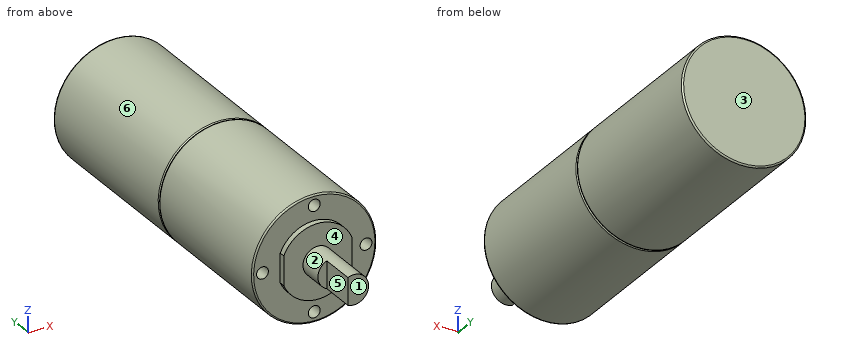
```python
from build123d import *

# Parameters (mm, degrees)
CROQUIS1_R              = 21
SALIENTE_EXTRUIR1_DEPTH = 60
REDONDEO1_R             = 0.5
SALIENTE_EXTRUIR2_START = 53
CROQUIS2_R              = 21
SALIENTE_EXTRUIR2_DEPTH = 53
REDONDEO2_R             = 0.5
SALIENTE_EXTRUIR3_DEPTH = 2
CROQUIS4_R              = 5
SALIENTE_EXTRUIR4_DEPTH = 20.5
CORTAR_EXTRUIR1_START   = -12
CORTAR_EXTRUIR1_DEPTH   = 12
CROQUIS6_R              = 2
CORTAR_EXTRUIR2_DEPTH   = 5


with BuildPart() as part:
    # Croquis1 → Saliente-Extruir1 (new body)
    with BuildSketch(Plane(origin=(0, 0, 0), x_dir=(1, 0, 0), z_dir=(0, 1, 0))):
        with Locations(Location((0, 0, 0), (0, 0, 270))):
            Circle(CROQUIS1_R)
    extrude(amount=SALIENTE_EXTRUIR1_DEPTH)

    # Redondeo1
    redondeo1_edges = [part.edges().sort_by_distance(p)[0] for p in [
        (0, 0, -21),
        (0, 60, -21),
    ]]
    fillet(redondeo1_edges, radius=REDONDEO1_R)

    # Croquis2 → Saliente-Extruir2 (add)
    with BuildSketch(Plane.XZ.offset(SALIENTE_EXTRUIR2_START)):
        with Locations(Location((0, 0, 0), (0, 0, 90))):
            Circle(CROQUIS2_R)
    extrude(amount=-SALIENTE_EXTRUIR2_DEPTH)

    # Redondeo2
    redondeo2_edges = [part.edges().sort_by_distance(p)[0] for p in [
        (0, 0, -21),
        (0, -53, -21),
    ]]
    fillet(redondeo2_edges, radius=REDONDEO2_R - 0.0001)  # a hair under: the kernel refuses the full size

    # Croquis3 → Saliente-Extruir3 (add)
    with BuildSketch(Plane.XZ.offset(53)):
        with BuildLine():
            Line((11.5, -4.898979486), (11.5, 4.898979486))
            ThreePointArc((11.5, 4.898979486), (0, 12.5), (-11.5, 4.898979486))
            Line((-11.5, 4.898979486), (-11.5, -4.898979486))
            ThreePointArc((-11.5, -4.898979486), (0, -12.5), (11.5, -4.898979486))
        make_face()
    extrude(amount=SALIENTE_EXTRUIR3_DEPTH)

    # Croquis4 → Saliente-Extruir4 (add)
    with BuildSketch(Plane.XZ.offset(55)):
        with Locations(Location((0, 0, 0), (0, 0, 270))):
            Circle(CROQUIS4_R)
    extrude(amount=SALIENTE_EXTRUIR4_DEPTH)

    # Croquis5 → Cortar-Extruir1 (cut)
    with BuildSketch(Plane.XZ.offset(75.5).offset(CORTAR_EXTRUIR1_START)):
        with BuildLine():
            Line((-2, 4.582575695), (-2, -4.582575695))
            ThreePointArc((-2, -4.582575695), (-5, 0), (-2, 4.582575695))
        make_face()
    extrude(amount=CORTAR_EXTRUIR1_DEPTH, mode=Mode.SUBTRACT)

    # Croquis6 → Cortar-Extruir2 (cut)
    with BuildSketch(Plane.XZ.offset(53)):
        with Locations(Location((-17.5, 0, 0), (0, 0, 270))):
            Circle(CROQUIS6_R)
        with Locations(Location((0, 17.5, 0), (0, 0, 270))):
            Circle(CROQUIS6_R)
        with Locations(Location((17.5, 0, 0), (0, 0, 270))):
            Circle(CROQUIS6_R)
        with Locations(Location((0, -17.5, 0), (0, 0, 270))):
            Circle(CROQUIS6_R)
    extrude(amount=-CORTAR_EXTRUIR2_DEPTH, mode=Mode.SUBTRACT)


solid = part.part
```
Could you check a few things on this model? Use its own coordinates, in mm. Face numbers are marked on the shaded views. A direction names the side the tool comes from. Round coordinates to 2 decimals unless told otherwise and drop trailing zeros. Order: outer loops, then holes, each group sorted by start corner. A loop starts at its lowest first (then second) coordinate and runs counter-clockwise, first axis right, second up. Notation, with made-up numbers: M 60.5,46 L 81.5,46 A29 cw 81.5,78 Z; hole C 38,22.25 d5. An arc over 180 degrees is marked long. One line per question, with ' | ' between items. Start each with the question number.
(1) Please list where these lines run through material, in increasing order: line 1 along X through (y, z) = (-49.65, 0); line 2 along Y through (x, z) = (-12, -16); line 3 along Y through (x, z) = (0, -11.5).
(2) For the marked faces 4, 5 and 6, which set-ups out of +Z, -Z, +X, -X, +Y, -Y let a thin tool reach every point of the face, with its end or its side?
(3) Suppose I cut it at D-D on y = -59. List the corners of the cut face in (x, z) for me.
(4) For P1, Ø1.5, axis at x = -16, y = -24.5, coming from the -Z side; P2, Ø4.5, axis at x = -17.5, z = 0, coming from the -Y side; P3, Ø0.9, axis at x = -4, z = -0.5, coming from the -Y side; P4, Ø12, axis at x = 1.5, y = -22, coming from the +Z side, each with a flat end and sliding along its axis, tell me the tip position at first contact or that it passes through.
(5) Thinking about a two-plate mould opening in Y: for the marked faces 1, 2 and 3, which applies, +Y half, -Y half, draft (parallel to the pull), parting line (faces both ways), or undercut?
(6) Suppose I cut it at C-C on y = 5. List the corners of the cut face in (x, z) for me.
Geometry results:
1) line 1: -21 to -19.5, -15.5 to 15.5, 19.5 to 21 | line 2: -53 to 60 | line 3: -55 to 60
2) face 4: -Y | face 5: +Z, -Z, -X, -Y | face 6: +Y, -Y
3) outline: C 0,0 d10
4) P1: z = -14.44 | P2: y = -53 | P3: y = -63.5 | P4: z = 21
5) face 1: -Y half | face 2: draft | face 3: +Y half
6) outline: C 0,0 d42
